Read the model definition and answer for the solid it produces. Units are mm, in the model's axes. Face numbers are marked on the shaded views. A direction names the side the tool comes from. Coordinates: 2 decimals unless noted, no trailing zeros. Write each loop counter-clockwise with the first axis right and the second up, starting at its lowest first coordinate (ties: lowest second). Pieces come first, ordered by that corner, then holes. Notation, with made-up numbers: (-8, -39) -> (13, -39) arc R25 cw to (13, -2) -> close; hole circle Ø3 at (30, 62.5). An arc over 180 degrees is marked (long way). Use CSV: the item, a comma, the result in double quotes.
from build123d import *

# Parameters (mm, degrees)
CROQUIS1_W              = 40
CROQUIS1_H              = 88
CROQUIS1_R              = 1.6
SALIENTE_EXTRUIR1_DEPTH = 18
CROQUIS3_W              = 40
CROQUIS3_H              = 74
CORTAR_EXTRUIR1_DEPTH   = 16
CROQUIS4_W              = 4
CROQUIS4_H              = 55.4
SALIENTE_EXTRUIR2_DEPTH = 6
CORTAR_EXTRUIR2_START   = -2
CORTAR_EXTRUIR2_DEPTH   = 51.4
CORTAR_EXTRUIR3_REACH   = 94.022
CROQUIS6_R              = 5.25
CHAFL_N1_SIZE           = 1
CORTAR_EXTRUIR4_DEPTH   = 1
CHAFL_N2_SIZE           = 1
CROQUIS8_R              = 2.8
CORTAR_EXTRUIR5_DEPTH   = 3.5


with BuildPart() as part:
    # Croquis1 → Saliente-Extruir1 (new body)
    with BuildSketch(Plane(origin=(0, 0, 0), x_dir=(1, 0, 0), z_dir=(0, 1, 0))):
        Rectangle(CROQUIS1_W, CROQUIS1_H)
        with Locations(Location((-12, 40, 0), (0, 0, 270))):
            Circle(CROQUIS1_R, mode=Mode.SUBTRACT)
        with Locations(Location((12, 40, 0), (0, 0, 90))):
            Circle(CROQUIS1_R, mode=Mode.SUBTRACT)
        with Locations(Location((-12, -40, 0), (0, 0, 90))):
            Circle(CROQUIS1_R, mode=Mode.SUBTRACT)
        with Locations(Location((12, -40, 0), (0, 0, 270))):
            Circle(CROQUIS1_R, mode=Mode.SUBTRACT)
    extrude(amount=SALIENTE_EXTRUIR1_DEPTH)

    # Croquis3 → Cortar-Extruir1 (cut)
    with BuildSketch(Plane(origin=(0, 18, 0), x_dir=(1, 0, 0), z_dir=(0, 1, 0))):
        Rectangle(CROQUIS3_W, CROQUIS3_H)
    extrude(amount=-CORTAR_EXTRUIR1_DEPTH, mode=Mode.SUBTRACT)

    # Croquis4 → Saliente-Extruir2 (add)
    with BuildSketch(Plane(origin=(0, 2, 0), x_dir=(1, 0, 0), z_dir=(0, 1, 0))):
        with Locations((-13.8, -1.7)):
            Rectangle(CROQUIS4_W, CROQUIS4_H)
    saliente_extruir2 = extrude(amount=SALIENTE_EXTRUIR2_DEPTH)

    # Croquis5 → Cortar-Extruir2 (cut)
    with BuildSketch(Plane.XY.offset(29.4).offset(CORTAR_EXTRUIR2_START)):
        Polygon((-11.8, 4), (-13, 4), (-13, 5.6), (-11.8, 6.8), align=None)
    cortar_extruir2 = extrude(amount=-CORTAR_EXTRUIR2_DEPTH, mode=Mode.SUBTRACT)

    # Simetría1: Saliente-Extruir2, Cortar-Extruir2 across plane
    add(saliente_extruir2.mirror(Plane(origin=(-1.4, 0, 0), x_dir=(0, 0, 1), z_dir=(1, 0, 0))))
    add(cortar_extruir2.mirror(Plane(origin=(-1.4, 0, 0), x_dir=(0, 0, 1), z_dir=(1, 0, 0))), mode=Mode.SUBTRACT)

    # Croquis6 → Cortar-Extruir3 (cut, up to next)
    with BuildSketch(Plane(origin=(0, 0, -44), x_dir=(-1, 0, 0), z_dir=(0, 0, -1)), mode=Mode.PRIVATE) as cortar_extruir3_sk1:
        with Locations((-5, 12.5)):
            Circle(CROQUIS6_R)
    cortar_extruir3_tool1 = extrude(cortar_extruir3_sk1.sketch, amount=-CORTAR_EXTRUIR3_REACH, mode=Mode.PRIVATE) & part.part
    add(cortar_extruir3_tool1.solids().sort_by_distance((5, 12.5, -44))[0], mode=Mode.SUBTRACT)

    # Chaflán1
    chafl_n1_edges = [part.edges().sort_by_distance(p)[0] for p in [
        (-15.8, 2, 1.7),
        (-15.8, 8, 1.7),
        (-11.8, 8, 1.7),
        (13, 8, 1.7),
        (9, 8, 1.7),
        (13, 2, 1.7),
    ]]
    chamfer(chafl_n1_edges, length=CHAFL_N1_SIZE)

    # Croquis7 → Cortar-Extruir4 (cut)
    with BuildSketch(Plane(origin=(0, 0, -44), x_dir=(-1, 0, 0), z_dir=(0, 0, -1))):
        Polygon((13.349277552, 10.843260825), (12.702142135, 10.843260825), (12.702142135, 14.343260825), (13.016244699, 14.343260825), (13.016244699, 11.202235184), (13.554706238, 11.202235184), align=None)
        with BuildLine():
            Line((10.952142135, 11.920183902), (11.266244699, 11.920183902))
            add(Edge.make_bspline(
                [(11.266244699, 11.920183902), (11.264197895, 11.878512809), (11.260178025, 11.796671891), (11.241344805, 11.677350891), (11.214421773, 11.563285573), (11.176265555, 11.455453837), (11.12914596, 11.352567543), (11.07145794, 11.255992901), (11.004431311, 11.16477142), (10.928189034, 11.080630224), (10.845459137, 11.003714652), (10.756737301, 10.936591237), (10.662935418, 10.880527385), (10.564867085, 10.833404425), (10.461398114, 10.79807587), (10.353517551, 10.771851148), (10.240737789, 10.756075643), (10.163897853, 10.754379741), (10.124818417, 10.753517236)],
                knots=[0, 0, 0, 0, 1.100776268, 2.161895295, 3.184016182, 4.190939212, 5.176500551, 6.166955529, 7.155448256, 8.160289653, 9.16017456, 10.133824356, 11.091467644, 12.04088621, 13.000931625, 13.972173743, 14.968683325, 16, 16, 16, 16], degree=3))
            add(Edge.make_bspline(
                [(10.124818417, 10.753517236), (10.086437642, 10.754408401), (10.01102079, 10.756159509), (9.900996983, 10.771423682), (9.796007884, 10.794814665), (9.697243334, 10.829476418), (9.60368973, 10.872969336), (9.516505422, 10.927058477), (9.433582202, 10.989184526), (9.358989797, 11.062465248), (9.290467674, 11.140655962), (9.231405748, 11.224162988), (9.180541152, 11.310511825), (9.138910069, 11.400376981), (9.107351857, 11.494051102), (9.083970246, 11.590636102), (9.070604054, 11.691246638), (9.068563952, 11.759355152), (9.06752675, 11.793981979)],
                knots=[0, 0, 0, 0, 1.111674182, 2.184400057, 3.212814286, 4.223731311, 5.211378316, 6.196328225, 7.191884489, 8.207283132, 9.220262353, 10.201199469, 11.166417575, 12.120932471, 13.06540007, 14.026332106, 14.996573967, 16, 16, 16, 16], degree=3))
            add(Edge.make_bspline(
                [(9.06752675, 11.793981979), (9.06922004, 11.842729793), (9.072576904, 11.939369965), (9.10129089, 12.081385135), (9.146138886, 12.218977383), (9.200131458, 12.32971846), (9.254614612, 12.418943506), (9.303662739, 12.492443272), (9.36140823, 12.571561933), (9.427357734, 12.656619722), (9.502646994, 12.746502735), (9.585320007, 12.843044827), (9.67751183, 12.944460868), (9.742160462, 13.013774517), (9.775659763, 13.049691114)],
                knots=[0, 0, 0, 0, 1.184416499, 2.348048165, 3.509039915, 4.696071444, 5.333504901, 6.05069495, 6.844171097, 7.714965912, 8.667477798, 9.695072654, 10.805644396, 12, 12, 12, 12], degree=3))
            Line((9.775659763, 13.049691114), (10.651360885, 13.984286466))
            Line((10.651360885, 13.984286466), (9.022654955, 13.984286466))
            Line((9.022654955, 13.984286466), (9.022654955, 14.343260825))
            Line((9.022654955, 14.343260825), (11.400860084, 14.343260825))
            Line((11.400860084, 14.343260825), (10.043488289, 12.894743197))
            add(Edge.make_bspline(
                [(10.043488289, 12.894743197), (10.010438062, 12.860246772), (9.946955341, 12.7939862), (9.857203547, 12.697218484), (9.776462338, 12.607551149), (9.704678153, 12.524586855), (9.641791929, 12.448795933), (9.588004874, 12.379584429), (9.543079259, 12.317546294), (9.495467468, 12.244666486), (9.450066467, 12.155578956), (9.410163632, 12.047256962), (9.386006998, 11.935501368), (9.383094384, 11.860003118), (9.381629314, 11.822026851)],
                knots=[0, 0, 0, 0, 1.329530082, 2.553755191, 3.672934919, 4.687409497, 5.60679272, 6.413407421, 7.126401618, 7.737995624, 8.834647426, 9.90044882, 10.943907757, 12, 12, 12, 12], degree=3))
            add(Edge.make_bspline(
                [(9.381629314, 11.822026851), (9.382258526, 11.798142814), (9.383498582, 11.751071962), (9.394649978, 11.682104068), (9.411033592, 11.615318538), (9.436285803, 11.551541126), (9.466625403, 11.489517454), (9.505386481, 11.431133235), (9.549680213, 11.374398292), (9.601058771, 11.321258018), (9.65746288, 11.272573276), (9.717059065, 11.229450114), (9.780108664, 11.193410762), (9.846348922, 11.16386733), (9.915594355, 11.140691931), (9.98797911, 11.124633356), (10.063303123, 11.114550871), (10.114736619, 11.113186699), (10.140944218, 11.112491595)],
                knots=[0, 0, 0, 0, 0.991504627, 1.954065223, 2.895985987, 3.842598665, 4.797835564, 5.759220273, 6.74786863, 7.784730864, 8.824135544, 9.839918996, 10.835834653, 11.835434876, 12.84861661, 13.863796685, 14.911511676, 16, 16, 16, 16], degree=3))
            add(Edge.make_bspline(
                [(10.140944218, 11.112491595), (10.168322043, 11.113178196), (10.222087569, 11.114526567), (10.300857634, 11.124746109), (10.376527654, 11.140223083), (10.447931577, 11.1648623), (10.516563758, 11.193699284), (10.580673358, 11.231038105), (10.642061294, 11.273703483), (10.699493344, 11.323448604), (10.75180153, 11.379603353), (10.799386756, 11.440726805), (10.839706189, 11.507902554), (10.875497343, 11.5795187), (10.90287051, 11.657542834), (10.926272606, 11.740066779), (10.943271549, 11.82826796), (10.949136163, 11.889036378), (10.952142135, 11.920183902)],
                knots=[0, 0, 0, 0, 1.031072318, 2.024855787, 2.988461151, 3.935103592, 4.865765533, 5.788564469, 6.724086513, 7.67908574, 8.64457978, 9.611397706, 10.591395687, 11.591555111, 12.622101007, 13.700900657, 14.821571223, 16, 16, 16, 16], degree=3))
        make_face()
        Polygon((8.663680597, 10.843260825), (8.327142135, 10.843260825), (7.160475468, 13.601473966), (5.993808802, 10.843260825), (5.65727034, 10.843260825), (7.138039571, 14.343260825), (7.182911366, 14.343260825), align=None)
    extrude(amount=-CORTAR_EXTRUIR4_DEPTH, mode=Mode.SUBTRACT)

    # Chaflán2
    chafl_n2_edges = [part.edges().sort_by_distance(p)[0] for p in [
        (0, 0, 44),
        (0, 0, -44),
    ]]
    chamfer(chafl_n2_edges, length=CHAFL_N2_SIZE)

    # Croquis8 → Cortar-Extruir5 (cut)
    with BuildSketch(Plane.XZ):
        with Locations(Location((-12, 40, 0), (0, 0, 270))):
            Circle(CROQUIS8_R)
        with Locations(Location((12, 40, 0), (0, 0, 270))):
            Circle(CROQUIS8_R)
        with Locations(Location((-12, -40, 0), (0, 0, 270))):
            Circle(CROQUIS8_R)
        with Locations(Location((12, -40, 0), (0, 0, 270))):
            Circle(CROQUIS8_R)
    extrude(amount=-CORTAR_EXTRUIR5_DEPTH, mode=Mode.SUBTRACT)


solid = part.part
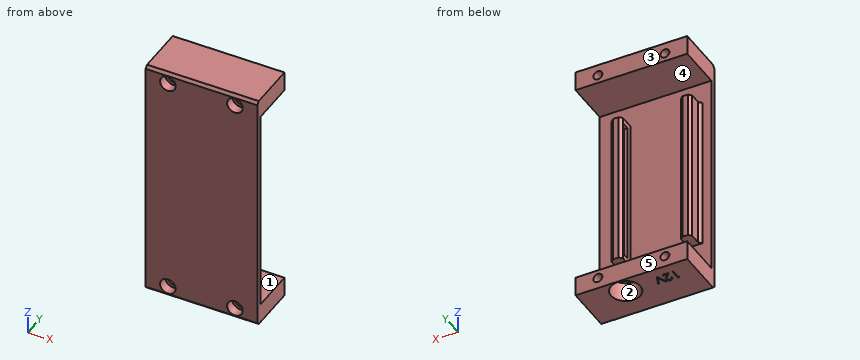
1. A cutting plane is placed at D-D (z = -23). Give the vertices of the cut face in (x, y).
Solutions:
outline,"(-20, 0) -> (20, 0) -> (20, 2) -> (14, 2) -> (13, 3) -> (13, 7) -> (12, 8) -> (10, 8) -> (9, 7) -> (9, 6.8) -> (10.2, 5.6) -> (10.2, 4) -> (9, 4) -> (9, 2) -> (-11.8, 2) -> (-11.8, 4) -> (-13, 4) -> (-13, 5.6) -> (-11.8, 6.8) -> (-11.8, 7) -> (-12.8, 8) -> (-14.8, 8) -> (-15.8, 7) -> (-15.8, 3) -> (-16.8, 2) -> (-20, 2) -> close"
2. A cutting plane is placed at B-B (z = 40). Give the vertices of the cut face in (x, y).
Solutions:
outline,"(-20, 0) -> (-14.8, 0) -> (-14.8, 3.5) -> (-13.6, 3.5) -> (-13.6, 18) -> (-20, 18) -> close; (-10.4, 3.5) -> (-9.2, 3.5) -> (-9.2, 0) -> (9.2, 0) -> (9.2, 3.5) -> (10.4, 3.5) -> (10.4, 18) -> (-10.4, 18) -> close; (13.6, 3.5) -> (14.8, 3.5) -> (14.8, 0) -> (20, 0) -> (20, 18) -> (13.6, 18) -> close"
3. For a pull along Y with two mould halves and no side action, classify the marked faces 1, 2 and 3 as pulls with the +Y half, pulls with the -Y half, needs draft (parallel to the pull), parting line crosses it, or undercut.
Solutions:
face 1,"needs draft"
face 2,"undercut"
face 3,"pulls with the +Y half"
4. A tool of negligible diameter and unlimited length cuts with its end or side. For the marked faces 4 and 5, from which of +Z, -Z, +X, -X, +Y, -Y can it reach the whole face along a straight path? Write none if from no direction.
Solutions:
face 4,"+X, -X, +Y"
face 5,"+Z, -Z, +X, -X, +Y"
5. Find the intervals of material crossed by line 1 along Z through (x, y) = (-12, 9); line 2 along X through (y, z) = (2.05, -40); line 3 along X through (y, z) = (13.25, 40), in increasing order.
Solutions:
line 1,"z = -44 to -41.6, -38.4 to -37, 37 to 38.4, 41.6 to 44"
line 2,"x = -20 to -14.8, -9.2 to 9.2, 14.8 to 20"
line 3,"x = -20 to -13.6, -10.4 to 10.4, 13.6 to 20"
6. A cutting plane is placed at A-A (x = 5). Give the vertices of the cut face in (y, z), and give its area (4 significant figures).
Solutions:
outline,"(0, -43) -> (1, -44) -> (7.25, -44) -> (7.25, -37) -> (2, -37) -> (2, 37) -> (18, 37) -> (18, 44) -> (1, 44) -> (0, 43) -> close; (17.75, -44) -> (18, -44) -> (18, -37) -> (17.75, -37) -> close"
area,"325.5 mm^2"
7. Each of these flat-tipped pins is pushed along its axis until it touches: pin 1 Ø0.6 at (x, z) = (-14, 7.5) entering from +Y; pin 2 Ø2 at (x, z) = (14, -33.5) entering from +Y; pin 3 Ø1.8 at (y, z) = (5, 5.5) entering from -X. Where does it stop, or does it pass through?
Solutions:
pin 1,"stops at y = 8"
pin 2,"stops at y = 2"
pin 3,"stops at x = -15.8"
8. A cutting plane is placed at C-C (y = 16). Give the vertices of the cut face in (x, z), and give its area (3 significant figures).
Solutions:
outline,"(-20, -44) -> (1.09, -44) -> (1.09, -37) -> (-20, -37) -> close; (-20, 37) -> (20, 37) -> (20, 44) -> (-20, 44) -> close; (8.91, -44) -> (20, -44) -> (20, -37) -> (8.91, -37) -> close; hole circle Ø3.2 at (-12, -40); hole circle Ø3.2 at (-12, 40); hole circle Ø3.2 at (12, -40); hole circle Ø3.2 at (12, 40)"
area,"473 mm^2"
